Check sheet for the drawn part. Datum: minimum x, y, z corner. Units: mm. Coordinates: 2 decimals unless noted, no trailing zeros. Order: outer loops, then holes, each group sorted by start corner. A loop starts at its lowest first (then second) coordinate and runs counter-clockwise, first axis right, second up. Notation, with made-up numbers: (-9, 4) -> (6, 4) arc R25 cw to (6, 29) -> close; hole circle Ø9 at (-11, 2). An arc over 180 degrees is marked (long way). Answer as CSV lines item,"result".
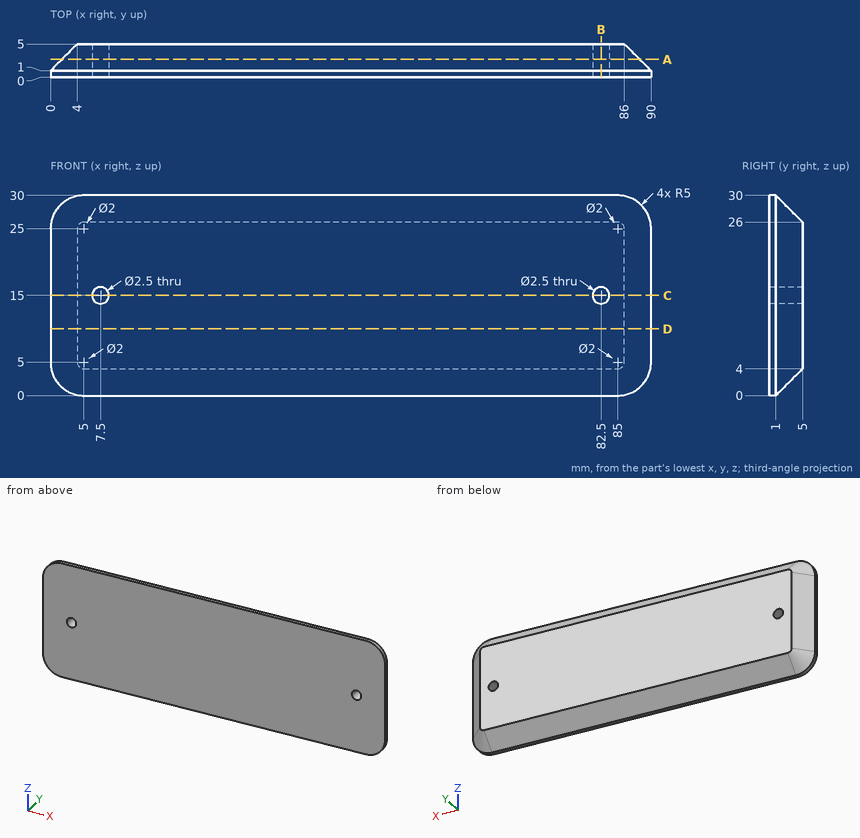
Item 1: Section check A-A, the plane y = 2.7. Record the boundary of the cut face in (x, z), plus the area to 3 significant figures.
Answer list:
outline,"(1.7, 5) arc R3.3 ccw to (5, 1.7) -> (85, 1.7) arc R3.3 ccw to (88.3, 5) -> (88.3, 25) arc R3.3 ccw to (85, 28.3) -> (5, 28.3) arc R3.3 ccw to (1.7, 25) -> close; hole circle Ø2.5 at (7.5, 15); hole circle Ø2.5 at (82.5, 15)"
area,"2,280 mm2"
Item 2: Thickness scan on line 1 (Y direction, x = 18, z = 27); line 2 (Z direction, x = 7.5, y = 3.2); line 3 (Z direction, x = 7.5, y = 1.6). Record the ranges inside material, lowest first.
Answer list:
line 1,"0 to 4"
line 2,"2.2 to 13.75, 16.25 to 27.8"
line 3,"0.6 to 13.75, 16.25 to 29.4"
Item 3: Section check C-C, the plane z = 15. Record the boundary of the cut face in (x, y), plus the area to 3 significant figures.
Answer list:
outline,"(0, 0) -> (6.25, 0) -> (6.25, 5) -> (4, 5) -> (0, 1) -> close; (8.75, 0) -> (81.25, 0) -> (81.25, 5) -> (8.75, 5) -> close; (83.75, 0) -> (90, 0) -> (90, 1) -> (86, 5) -> (83.75, 5) -> close"
area,"409 mm2"
Item 4: Depth check by flat-ended pin: pin 1 Ø6 at (x, z) = (67.5, 18.5) entering from -Y; pin 2 Ø3 at (y, z) = (4, 19.5) entering from +X. Enter the tip coordinate at first touch or a pass-through.
Answer list:
pin 1,"y = 0"
pin 2,"x = 88.5"
Item 5: Section check B-B, the plane x = 82.5. Record the boundary of the cut face in (y, z).
Answer list:
outline,"(0, 0) -> (1, 0) -> (5, 4) -> (5, 13.75) -> (0, 13.75) -> close; (0, 16.25) -> (5, 16.25) -> (5, 26) -> (1, 30) -> (0, 30) -> close"
Item 6: Section check D-D, the plane z = 10. Record the boundary of the cut face in (x, y).
Answer list:
outline,"(0, 0) -> (90, 0) -> (90, 1) -> (86, 5) -> (4, 5) -> (0, 1) -> close"
